```python
from build123d import *

# Parameters (mm, degrees)
SKETCH1_R           = 12.0269
BOSS_EXTRUDE1_DEPTH = 65.8876
SKETCH2_W           = 19.05
SKETCH2_H           = 3.175
BOSS_EXTRUDE2_DEPTH = 23.0124
CUT_EXTRUDE1_DEPTH  = 14.6144


with BuildPart() as part:
    # Sketch1 → Boss-Extrude1 (new body)
    with BuildSketch(Plane(origin=(0, 0, 0), x_dir=(1, 0, 0), z_dir=(0, 1, 0))):
        Circle(SKETCH1_R)
    extrude(amount=BOSS_EXTRUDE1_DEPTH)

    # Sketch2 → Boss-Extrude2 (add)
    with BuildSketch(Plane(origin=(0, 65.8876, 0), x_dir=(1, 0, 0), z_dir=(0, 1, 0))):
        Rectangle(SKETCH2_W, SKETCH2_H)
    boss_extrude2 = extrude(amount=BOSS_EXTRUDE2_DEPTH)

    # Sketch3 → Cut-Extrude1 (cut, through all)
    with BuildSketch(Plane.XY.offset(1.5875)):
        with BuildLine():
            Line((-4.3688, 78.98511), (-4.3688, 78.1939))
            ThreePointArc((-4.3688, 78.1939), (0, 73.8251), (4.3688, 78.1939))
            Line((4.3688, 78.1939), (4.3688, 78.98511))
            ThreePointArc((4.3688, 78.98511), (0, 83.35391), (-4.3688, 78.98511))
        make_face()
    cut_extrude1 = extrude(amount=-CUT_EXTRUDE1_DEPTH, mode=Mode.SUBTRACT)

    # Mirror2: Boss-Extrude2, Cut-Extrude1 across plane
    add(boss_extrude2.mirror(Plane.ZX.offset(32.9438)))
    add(cut_extrude1.mirror(Plane.ZX.offset(32.9438)), mode=Mode.SUBTRACT)


solid = part.part
```
Read the model definition and answer for the solid it produces. Units are mm, in the model's axes. A direction names the side the tool comes from. Coordinates: 2 decimals unless noted, no trailing zeros. Loops run counter-clockwise (first coordinate to the right, second up) from the corner with the lowest first, then second, coordinate; pieces in that order, holes last. Notation, with made-up numbers: (28.25, 87.5) -> (51.25, 87.5) arc R28 cw to (51.25, 122.5) -> close; hole circle Ø6 at (-2, 9). An arc over 180 degrees is marked (long way). Return JSON: item names as keys, results as strings.
Item 1: Flat-ended cylindrical pins translate along their axes: P1, Ø10, axis at y = 69, z = -7.5, coming from the +X side; P2, Ø8, axis at y = 40.5, z = -0.5, coming from the +X side; P3, Ø0.9, axis at y = 78.5, z = 0.5, coming from the +X side (3 decimals); P4, Ø1.6, axis at y = 82.5, z = 0, coming from the -X side (3 decimals). Find the tip coordinate at first contact, or state that the pin passes through.
Answers:
{"P1": "stops at x = 11.48", "P2": "stops at x = 12.03", "P3": "stops at x = 9.525", "P4": "stops at x = -9.525"}
Item 2: For faces 1 (the flat face through (-9.525, -11, 0)), 2 (the cylindrical face through (0.096, -17.465, 0.022)), 3 (the flat face through (-4, -9, -1.588)), determine the directions among +Z, -Z, +X, -X, +Y, -Y from which every point of the face is accessible in a straight line to the end or side of a thin tool.
Answers:
{"face 1": "+Z, -Z, -X, -Y", "face 2": "+Z, -Z", "face 3": "-Z, +X, -X, -Y"}
Item 3: Find section B-B (z = 0). Determine the outline of the cut face in (x, y) (1 decimal).
Answers:
{"outline": "(-12, 0) -> (-9.5, 0) -> (-9.5, -23) -> (9.5, -23) -> (9.5, 0) -> (12, 0) -> (12, 65.9) -> (9.5, 65.9) -> (9.5, 88.9) -> (-9.5, 88.9) -> (-9.5, 65.9) -> (-12, 65.9) -> close; hole (-4.4, -13.1) arc R4.4 ccw to (4.4, -13.1) -> (4.4, -12.3) arc R4.4 ccw to (-4.4, -12.3) -> close; hole (-4.4, 78.2) arc R4.4 ccw to (4.4, 78.2) -> (4.4, 79) arc R4.4 ccw to (-4.4, 79) -> close"}
Item 4: Find section A-A (x = 0). Determine the outline of the cut face in (y, z), plus the area to 3 significant figures.
Answers:
{"outline": "(-23.01, -1.59) -> (-17.47, -1.59) -> (-17.47, 1.59) -> (-23.01, 1.59) -> close; (-7.94, -1.59) -> (0, -1.59) -> (0, -12.03) -> (65.89, -12.03) -> (65.89, -1.59) -> (73.83, -1.59) -> (73.83, 1.59) -> (65.89, 1.59) -> (65.89, 12.03) -> (0, 12.03) -> (0, 1.59) -> (-7.94, 1.59) -> close; (83.35, -1.59) -> (88.9, -1.59) -> (88.9, 1.59) -> (83.35, 1.59) -> close", "area": "1,670 mm2"}
Item 5: Find the intervals of material crossed by probe 1 along Y at (x, z) = (-0.25, 5.5); probe 2 along Z at (x, y) = (6.25, -16.5); probe 3 along Y at (x, z) = (-1, 0.75), in increasing order.
Answers:
{"probe 1": "y = 0 to 65.89", "probe 2": "z = -1.59 to 1.59", "probe 3": "y = -23.01 to -17.35, -8.05 to 73.94, 83.24 to 88.9"}
Item 6: Find section C-C (y = 82). Determine the outline of the cut face in (x, z) (1 decimal), plus the area to 3 significant figures.
Answers:
{"outline": "(-9.5, -1.6) -> (-3.2, -1.6) -> (-3.2, 1.6) -> (-9.5, 1.6) -> close; (3.2, -1.6) -> (9.5, -1.6) -> (9.5, 1.6) -> (3.2, 1.6) -> close", "area": "40.4 mm2"}
Item 7: Find section D-D (x = 6). Determine the outline of the cut face in (y, z), plus the area to 3 significant figures.
Answers:
{"outline": "(-23.01, -1.59) -> (0, -1.59) -> (0, -10.42) -> (65.89, -10.42) -> (65.89, -1.59) -> (88.9, -1.59) -> (88.9, 1.59) -> (65.89, 1.59) -> (65.89, 10.42) -> (0, 10.42) -> (0, 1.59) -> (-23.01, 1.59) -> close", "area": "1,520 mm2"}
Item 8: For a pull along X with two mould halves and no side action, classify faces 4 (the flat face through (-4, -9, 1.588)), 5 (the flat face through (9.525, 77, 0)), 6 (the cylindrical face through (0.096, 83.353, 0.022)), 7 (the flat face through (-9.525, 77, 0)) as +X half, -X half, draft (parallel to the pull), parting line (faces both ways), or undercut.
Answers:
{"face 4": "draft", "face 5": "+X half", "face 6": "undercut", "face 7": "-X half"}
